Verification items for the finished model (mm, model axes). Coordinates: 2 decimals unless noted, no trailing zeros. Order: outer loops, then holes, each group sorted by start corner. A loop starts at its lowest first (then second) coordinate and runs counter-clockwise, first axis right, second up. Notation, with made-up numbers: (20, 11) -> (62, 11) arc R17 ccw to (62, 27) -> close; hole circle Ø5 at (39.25, 38). An arc over 180 degrees is marked (long way). Use CSV: the item, a comma, the result in double quotes. Start each with the question number.
1) Sectioned sample at B-B on y = 0. Record the boundary of the cut face in (x, z).
2) Sectioned sample at C-C on x = 22. Record the boundary of the cut face in (y, z), then the cut area to 3 significant figures.
3) Go/stop test with flat-tipped pins: pin 1 (1.2 mm diameter, centred on y = -54, z = 2.5, fed in from +X); pin 2 (3 mm diameter, centred on x = 19, y = 2.5, fed in from -Z); pin 3 (2 mm diameter, centred on x = -13.5, y = -30, fed in from +Z); pin 4 (1 mm diameter, centred on x = -24, z = 0.5, fed in from -Y). Record where each tip stops, or that it passes through.
4) Scan lines: line 1 along X through (y, z) = (13.5, 0.3); line 2 along Z through (x, y) = (44, -0.5); line 3 along Y through (x, z) = (-7, 1.2). Record each from-to range of solid material in increasing order.
5) Sectioned sample at A-A on z = 1.05. Record the boundary of the cut face in (x, y) (3 decimals).
from build123d import *

# Parameters (mm, degrees)
SKETCH1_W           = 105.5
SKETCH1_H           = 75.06
BOSS_EXTRUDE1_DEPTH = 2
SKETCH2_W           = 7.5
SKETCH2_H           = 7.5
SKETCH2_R           = 1.125
BOSS_EXTRUDE2_DEPTH = 2
CUT_EXTRUDE1_START  = -4
SKETCH3_R           = 1.125
CUT_EXTRUDE1_DEPTH  = 4
SKETCH4_R           = 1.125
CUT_EXTRUDE2_DEPTH  = 4
SKETCH5_W           = 7.5
SKETCH5_H           = 7.5
BOSS_EXTRUDE3_DEPTH = 2
SKETCH6_R           = 1.125
CUT_EXTRUDE3_DEPTH  = 4
SKETCH7_W           = 7.5
SKETCH7_H           = 7.5
BOSS_EXTRUDE4_DEPTH = 2
SKETCH8_R           = 1.125
CUT_EXTRUDE4_DEPTH  = 4
FILLET2_R           = 1
FILLET3_R           = 1
CHAMFER1_SIZE       = 1


with BuildPart() as part:
    # Sketch1 → Boss-Extrude1 (new body)
    with BuildSketch(Plane.XY):
        with Locations((9.308823529, -13.027464503)):
            Rectangle(SKETCH1_W, SKETCH1_H)
    extrude(amount=BOSS_EXTRUDE1_DEPTH)

    # Sketch2 → Boss-Extrude2 (add)
    # profile 1 of 2: a face of its own
    with BuildSketch(Plane.XY.offset(2)):
        with Locations((58.308823529, -46.807464503)):
            Rectangle(SKETCH2_W, SKETCH2_H)
    # profile 2 of 2: a face of its own
    with BuildSketch(Plane.XY.offset(2)):
        with Locations((58.308823529, 20.752535497)):
            Rectangle(SKETCH2_W, SKETCH2_H)
        with Locations((58.308823529, 20.752535497)):
            Circle(SKETCH2_R, mode=Mode.SUBTRACT)
    extrude(amount=BOSS_EXTRUDE2_DEPTH)

    # Sketch3 → Cut-Extrude1 (cut)
    with BuildSketch(Plane.XY.offset(2).offset(CUT_EXTRUDE1_START)):
        with Locations((58.308823529, 20.752535497)):
            Circle(SKETCH3_R)
    extrude(amount=CUT_EXTRUDE1_DEPTH, mode=Mode.SUBTRACT)

    # Sketch4 → Cut-Extrude2 (cut)
    with BuildSketch(Plane.XY.offset(4)):
        with Locations((58.308823529, -46.807464503)):
            Circle(SKETCH4_R)
    extrude(amount=-CUT_EXTRUDE2_DEPTH, mode=Mode.SUBTRACT)

    # Sketch5 → Boss-Extrude3 (add, symmetric)
    with BuildSketch(Plane.XY.offset(2)):
        with Locations((-47.191176471, 20.752535497)):
            Rectangle(SKETCH5_W, SKETCH5_H)
    extrude(amount=BOSS_EXTRUDE3_DEPTH, both=True)

    # Sketch6 → Cut-Extrude3 (cut)
    with BuildSketch(Plane.XY.offset(4)):
        with Locations((-47.191176471, 20.752535497)):
            Circle(SKETCH6_R)
    extrude(amount=-CUT_EXTRUDE3_DEPTH, mode=Mode.SUBTRACT)

    # Sketch7 → Boss-Extrude4 (add, symmetric)
    with BuildSketch(Plane.XY.offset(2)):
        with Locations((-39.691176471, -54.307464503)):
            Rectangle(SKETCH7_W, SKETCH7_H)
    extrude(amount=BOSS_EXTRUDE4_DEPTH, both=True)

    # Sketch8 → Cut-Extrude4 (cut)
    with BuildSketch(Plane.XY.offset(4)):
        with Locations((-39.691176471, -54.307464503)):
            Circle(SKETCH8_R)
    extrude(amount=-CUT_EXTRUDE4_DEPTH, mode=Mode.SUBTRACT)

    # Fillet2
    fillet2_edges = [part.edges().sort_by_distance(p)[0] for p in [
        (-39.691176471, -50.557464503, 2),
        (-43.441176471, 20.752535497, 2),
    ]]
    fillet(fillet2_edges, radius=FILLET2_R)

    # Fillet3
    fillet3_edges = [part.edges().sort_by_distance(p)[0] for p in [
        (54.558823529, 20.752535497, 2),
        (58.308823529, 17.002535497, 2),
        (54.558823529, -46.807464503, 2),
        (58.308823529, -43.057464503, 2),
    ]]
    fillet(fillet3_edges, radius=FILLET3_R)

    # Chamfer1
    chamfer1_edges = [part.edges().sort_by_distance(p)[0] for p in [
        (-50.941176471, 24.502535497, 2),
        (-43.441176471, -58.057464503, 2),
        (62.058823529, 24.502535497, 2),
        (62.058823529, -50.557464503, 2),
    ]]
    chamfer(chamfer1_edges, length=CHAMFER1_SIZE)


solid = part.part
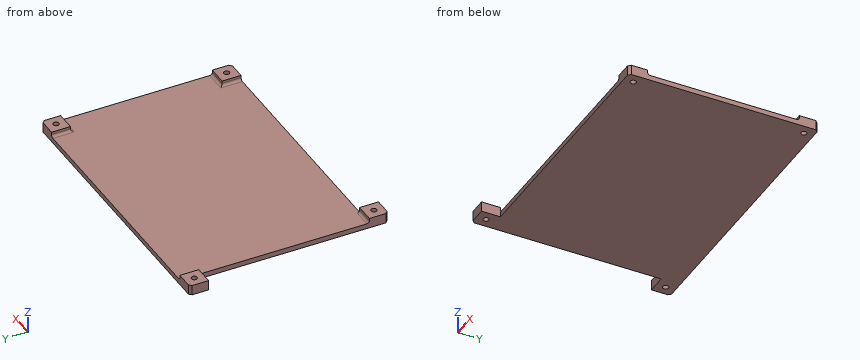
Answers follow:
1,outline,"(-43.44, 0) -> (62.06, 0) -> (62.06, 2) -> (-43.44, 2) -> close"
2,outline,"(-50.56, 0) -> (24.5, 0) -> (24.5, 2) -> (-50.56, 2) -> close"
2,area,"150 mm²"
3,pin 1,"stops at x = -35.94"
3,pin 2,"stops at z = 0"
3,pin 3,"stops at z = 2"
3,pin 4,"stops at y = -50.56"
4,line 1,"x = -43.44 to 62.06"
4,line 2,"z = 0 to 2"
4,line 3,"y = -50.56 to 24.5"
5,outline,"(-50.941, 17.003) -> (-43.441, 17.003) -> (-43.441, -57.057) -> (-42.441, -58.057) -> (-35.941, -58.057) -> (-35.941, -50.557) -> (61.059, -50.557) -> (62.059, -49.557) -> (62.059, 23.503) -> (61.059, 24.503) -> (-49.941, 24.503) -> (-50.941, 23.503) -> close; hole circle Ø2.25 at (-47.191, 20.753); hole circle Ø2.25 at (-39.691, -54.307); hole circle Ø2.25 at (58.309, -46.807); hole circle Ø2.25 at (58.309, 20.753)"
